from build123d import *

# Parameters (mm, degrees)
F0_W     = 81.09111
F0_H     = 119.011938
F0_R     = 2.5
F0_R_2   = 1.35255
F0_R_3   = 1.6
F0_R_4   = 5.969
F1_DEPTH = 1.70942
F2_R     = 5.674995


with BuildPart() as f1:
    # F0 (on Top) → F1 (new body)
    with BuildSketch(Plane.XY):
        Rectangle(F0_W, F0_H)
        with Locations((-34.870555, -53.830969)):
            Circle(F0_R, mode=Mode.SUBTRACT)
        with Locations((-27.80665, -50.137809)):
            Circle(F0_R_2, mode=Mode.SUBTRACT)
        with Locations((-27.80665, -28.749815)):
            Circle(F0_R_2, mode=Mode.SUBTRACT)
        with Locations((27.80665, -50.137809)):
            Circle(F0_R_2, mode=Mode.SUBTRACT)
        with Locations((34.870555, -53.830969)):
            Circle(F0_R, mode=Mode.SUBTRACT)
        with Locations((27.80665, -28.749815)):
            Circle(F0_R_2, mode=Mode.SUBTRACT)
        with Locations((-34.870555, 53.830969)):
            Circle(F0_R, mode=Mode.SUBTRACT)
        with Locations((-15.494, 41.344969)):
            Circle(F0_R_3, mode=Mode.SUBTRACT)
        with Locations((-7.747, 54.763167)):
            Circle(F0_R_3, mode=Mode.SUBTRACT)
        with Locations((0, 33.978969)):
            Circle(F0_R_4, mode=Mode.SUBTRACT)
        with Locations((15.494, 41.344969)):
            Circle(F0_R_3, mode=Mode.SUBTRACT)
        with Locations((7.747, 54.763167)):
            Circle(F0_R_3, mode=Mode.SUBTRACT)
        with Locations((34.870555, 53.830969)):
            Circle(F0_R, mode=Mode.SUBTRACT)
    extrude(amount=F1_DEPTH)

    # F2
    f2_edges = [f1.edges().sort_by_distance(p)[0] for p in [
        (40.545555, 59.505969, 0.85471),
        (40.545555, -59.505969, 0.85471),
        (-40.545555, -59.505969, 0.85471),
        (-40.545555, 59.505969, 0.85471),
    ]]
    fillet(f2_edges, radius=F2_R)


solid = f1.part
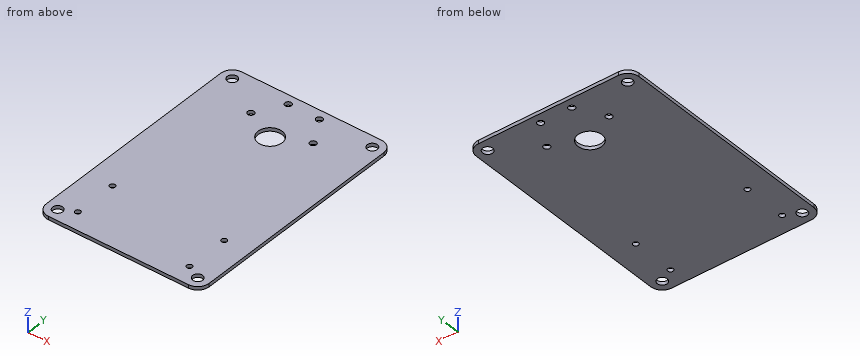
Source: CAD feature listing. Evaluate the final solid. Frame: model axes, mm. Give positions to 0.01 mm unless a question says otherwise; leave off trailing zeros. Write each loop counter-clockwise with the first axis right and the second up, starting at its lowest first coordinate (ties: lowest second). Pieces come first, ordered by that corner, then holes. Notation, with made-up numbers: (-23, -10.5) - (23, -10.5) arc R30 cw to (23, 18.5) - close; hole circle Ø3 at (-3, -33). An arc over 180 degrees is marked (long way). Write item = value, one per line. Start each with the question number.
Q1. Cut plane B-B, the plane z = 0.3. Give the number of separate pieces and of enclosed holes in the cut face, then the cut area to 3 significant figures.
Q2. Cut plane A-A, the plane x = 0. Return loops of the section in (y, z), then the cut area to 3 significant figures.
Q3. Material intervals for probe 1 along Y at (x, z) = (-15.5, 0.6); probe 2 along X at (y, z) = (-53, 0.9); probe 3 along X at (y, z) = (35, 0.55), sorted ascending.
Computed values:
q1.separate_pieces = 1
q1.enclosed_holes = 13
q1.area = 9,380 mm²
q2.outline = (-59.51, 0) - (28.01, 0) - (28.01, 1.71) - (-59.51, 1.71) - close; (39.95, 0) - (59.51, 0) - (59.51, 1.71) - (39.95, 1.71) - close
q2.area = 183 mm²
q3.probe_1 = -59.51 to 39.74, 42.94 to 59.51
q3.probe_2 = -40.55 to -37.23, -32.51 to 32.51, 37.23 to 40.55
q3.probe_3 = -40.55 to -5.88, 5.88 to 40.55
